Geometry check sheet. Reference: the model listing, model coordinates, mm. A direction names the side the tool comes from. Give positions to 0.01 mm unless a question says otherwise; leave off trailing zeros. Write each loop counter-clockwise with the first axis right and the second up, starting at its lowest first coordinate (ties: lowest second). Pieces come first, ordered by that corner, then holes. Notation, with made-up numbers: (13, 4) - (37, 4) arc R19 cw to (37, 19) - close; hole circle Ø3 at (-11, 77). An arc over 180 degrees is marked (long way). Write item = value, one per line. Start each with the question number.
(1) Draft check along Y on faces 1 (the cylindrical face through (4.085, 0.881, 7.386)), 2 (the cylindrical face through (4.853, -0.009, 7.414)), 3 (the cylindrical face through (-6.122, 0.377, 7.414)), 4 (the flat face through (-8, -21.8, 4)). Enter one of: pulls with the +Y half, pulls with the -Y half, needs draft (parallel to the pull), parting line crosses it, or undercut.
(2) Section check D-D, the plane y = -17.5. Enter the section's corners in (x, z).
(3) Section check B-B, the plane z = 7.75. Enter the section's corners in (x, y).
(4) Thickness scan on L1, parallel to Y at x = -6, z = 7.7; L2, parallel to Y at x = -6, z = 3.75; L3, parallel to Y at x = -6, z = 6.25. Record the ranges inside material, lowest first.
(5) Section check A-A, the plane z = 4.25. Enter the section's corners in (x, y).
(6) Section check C-C, the plane x = -10. Enter the section's corners in (y, z), plus the area to 3 significant figures.
(7) Access from +Z, -Z, +X, -X, +Y, -Y to the whole of each face (thin tool, end or side, straight path). Record for faces 5 (the flat face through (-5, -19, 5.4)), 6 (the flat face through (-6, 15.424, 3)), 7 (the flat face through (-11.646, -15.674, 5.192)).
(8) Depth check by flat-ended pin: pin 1 Ø4.5 at (x, y) = (-6, 17.5) entering from +Z; pin 2 Ø3.5 at (x, y) = (-6, -17.5) entering from -Z; pin 3 Ø1.5 at (y, z) = (14.5, 5.5) entering from +X; pin 4 Ø5 at (x, y) = (-4.5, 2.5) entering from -Z. Enter the tip coordinate at first touch or a pass-through.
Autodesk Inventor part; units mm, degrees
ref_plane "YZ Plane" through (0, 0, 0) normal (1, 0, 0) x (0, 1, 0)
ref_plane "XZ Plane" through (0, 0, 0) normal (0, 1, 0) x (-1, 0, 0)
ref_plane "XY Plane" through (0, 0, 0) normal (0, 0, 1) x (1, 0, 0)
sketch "Sketch1" plane through (0, 0, 0) normal (0, 0, 1) x (1, 0, 0)
  circle A0 centre (1.9608, 0) radius 2 construction
  circle A1 centre (-6, -17.5) radius 1.5 construction
  circle A2 centre (-6, 17.5) radius 1.5 construction
  line L0 (11.3072, 21.8) -> (-13.8, 21.8) construction
  line L1 (-13.8, 21.8) -> (-13.8, -21.8) construction
  line L2 (-13.8, -21.8) -> (11.3072, -21.8) construction
  line L3 (11.3072, -21.8) -> (11.3072, 21.8) construction
  line L4 (-18.8214, 0) -> (16.3286, 0) construction
  line L5 (-2.5075, 14.4235) -> (-13.8, 14.4235) construction
  circle A3 centre (-6, -17.5) radius 1.5 construction
  line L6 (11.3072, -21.8) -> (-13.8, -21.8) construction
  line L7 (-13.8, -21.8) -> (11.3072, -21.8)
  line L8 (-2.5075, -14.4235) -> (-13.8, -14.4235) construction
  circle A4 centre (-6, 17.5) radius 1.6
  circle A5 centre (-6, -17.5) radius 1.6
  line L9 (-13.8, 21.8) -> (11.3072, 21.8)
  line L10 (11.3072, 21.8) -> (11.3072, 15.4235)
  line L11 (11.3072, 15.4235) -> (-13.8, 15.4235)
  line L12 (-13.8, 15.4235) -> (-13.8, 21.8)
  line L13 (11.3072, 21.8) -> (11.3072, -21.8) construction
  line L14 (-13.8, -21.8) -> (11.3072, -21.8)
  line L15 (11.3072, -21.8) -> (11.3072, -15.4235)
  line L16 (11.3072, -15.4235) -> (-13.8, -15.4235)
  line L17 (-13.8, -15.4235) -> (-13.8, -21.8)
  point P0 (0, 0)
  dimension "d0" = 0.1
  dimension "d1" = 0.1
  dimension "d13" = 1
extrude "Extrusion1" add sketch "Sketch1" along normal blind 6.4
sketch "Sketch2" plane through (0, 0, 6.4) normal (0, 0, 1) x (1, 0, 0)
  circle A0 centre (-6, 17.5) radius 1.6 construction
  circle A1 centre (-6, -17.5) radius 1.6 construction
  line L0 (11.3072, 21.8) -> (-13.8, 21.8)
  line L1 (-13.8, -21.8) -> (11.3072, -21.8)
  line L2 (-13.8, 21.8) -> (11.3072, 21.8)
  line L3 (11.3072, 21.8) -> (11.3072, -21.8)
  line L4 (11.3072, -21.8) -> (-13.8, -21.8)
  line L5 (-13.8, -21.8) -> (-13.8, 21.8)
  circle A2 centre (-6, -17.5) radius 1.7
  circle A3 centre (-6, 17.5) radius 1.7
  circle A4 centre (1.9608, 0) radius 2 construction
  circle A5 centre (1.9608, 0) radius 2.3
  line L6 (-2.9164, -21.8) -> (3.0965, -2)
  line L7 (3.0965, 2) -> (-2.9164, 21.8)
  line L8 (-13.8, 21.8) -> (11.3072, 21.8)
  point P0 (0, 0)
  dimension "d6" = 0.1
  dimension "d7" = 0.1
  dimension "d8" = 0.3
extrude "Extrusion2" add sketch "Sketch2" along normal blind 2 contours L3 L1 L6 A5 L7 L0 | L7 A5 L6 L1 L5 L0
sketch "Sketch3" plane through (0, 0, 8.4) normal (0, 0, 1) x (1, 0, 0)
  circle A0 centre (1.9608, 0) radius 2.3 construction
  circle A1 centre (-6, 17.5) radius 1.7 construction
  circle A2 centre (-6, -17.5) radius 1.7 construction
  line L0 (11.3072, 21.8) -> (-13.8, 21.8) construction
  line L1 (-13.8, 21.8) -> (-13.8, -21.8) construction
  line L2 (-13.8, -21.8) -> (11.3072, -21.8) construction
  line L3 (11.3072, -21.8) -> (11.3072, 21.8) construction
  circle A3 centre (-6, -17.5) radius 2.8
  circle A4 centre (-6, 17.5) radius 2.8
  point P0 (0, 0)
  dimension "d9" = 5.6
  dimension "d10" = 5.6
extrude "Extrusion3" cut sketch "Sketch3" against normal blind 3
sketch "Sketch4" plane through (0, 0, 8.4) normal (0, 0, 1) x (1, 0, 0)
  circle A0 centre (-6, -17.5) radius 2.8 construction
  circle A1 centre (-6, 17.5) radius 2.8 construction
  circle A2 centre (1.9608, 0) radius 2.3 construction
  line L0 (11.3072, 21.8) -> (-13.8, 21.8) construction
  line L1 (-13.8, 21.8) -> (-13.8, -21.8) construction
  line L2 (-13.8, -21.8) -> (11.3072, -21.8) construction
  line L3 (11.3072, -21.8) -> (11.3072, 21.8)
  line L4 (11.3072, -21.8) -> (11.3072, 21.8)
  line L5 (11.3072, 21.8) -> (-2.6928, 21.8)
  line L6 (-13.8, 21.8) -> (11.3072, 21.8)
  line L7 (-2.6928, 21.8) -> (4.7397, 0.6635)
  line L8 (4.7397, -0.6635) -> (-2.6928, -21.8)
  line L9 (-13.8, -21.8) -> (11.3072, -21.8)
  line L10 (-2.6928, -21.8) -> (11.3072, -21.8)
  line L11 (11.3072, -21.8) -> (11.3072, 21.8)
  arc A3 (4.7397, -0.6635) -> (4.7397, 0.6635) centre (2.853, 0) ccw
  line L12 (-13.8, 21.8) -> (-6.243, 1.0605)
  line L13 (-6.2354, -0.2877) -> (-13.8, -21.8)
  line L14 (-13.8, 21.8) -> (-13.8, -21.8)
  arc A4 (-6.2354, -0.2877) -> (-6.243, 1.0605) centre (-8.1221, 0.3758) ccw
  point P0 (4.973, 0)
  dimension "d14" = 14
  dimension "d17" = 2
  dimension "d18" = 2
extrude "Extrusion4" cut sketch "Sketch4" against normal through all contours L9 L8 A3 L7 L5 L3 | L14 L12 A4 L13
equation "\"d10\" = d9"
properties part number "20_focus_inlet_plate_top"
Model answer:
q1.face_1 = undercut
q1.face_2 = parting line crosses it
q1.face_3 = undercut
q1.face_4 = pulls with the -Y half
q2.outline = (-12.29, 0) - (-7.6, 0) - (-7.6, 5.4) - (-8.8, 5.4) - (-8.8, 8.4) - (-12.29, 8.4) - close; (-4.4, 0) - (-1.18, 0) - (-1.18, 8.4) - (-3.2, 8.4) - (-3.2, 5.4) - (-4.4, 5.4) - close
q3.outline = (-13.8, -21.8) - (-2.69, -21.8) - (4.74, -0.66) arc R2 ccw to (4.74, 0.66) - (-2.69, 21.8) - (-13.8, 21.8) - (-6.24, 1.06) arc R2 cw to (-6.24, -0.29) - close; hole circle Ø5.6 at (-6, -17.5); hole circle Ø5.6 at (-6, 17.5); hole circle Ø4.6 at (1.96, 0)
q4.L1 = -21.8 to -20.3, -14.7 to 14.7, 20.3 to 21.8
q4.L2 = -21.8 to -19.1, -15.9 to -15.42, 15.42 to 15.9, 19.1 to 21.8
q4.L3 = -21.8 to -20.3, 20.3 to 21.8
q5.outline = (-13.8, -21.8) - (-2.69, -21.8) - (-0.45, -15.42) - (-11.56, -15.42) - close; (-13.8, 21.8) - (-11.48, 15.42) - (-0.45, 15.42) - (-2.69, 21.8) - close; hole circle Ø3.2 at (-6, -17.5); hole circle Ø3.2 at (-6, 17.5)
q6.outline = (-21.8, 0) - (-15.42, 0) - (-15.42, 6.4) - (-10.99, 6.4) - (-10.99, 8.4) - (-21.8, 8.4) - close; (11.37, 6.4) - (15.42, 6.4) - (15.42, 0) - (21.8, 0) - (21.8, 8.4) - (11.37, 8.4) - close
q6.area = 124 mm²
q7.face_5 = +Z
q7.face_6 = -Z, +X, -X
q7.face_7 = +Z, -Z, -X
q8.pin_1 = 5.4
q8.pin_2 = 0
q8.pin_3 = through
q8.pin_4 = 6.4
